The drawing under review shows one solid part. Ordinate dimensions are in mm from its lowest x, y, z. Give positions to 0.01 mm unless a question says otherwise; leave off trailing zeros. Order: outer loops, then holes, each group sorted by start corner. A loop starts at its lowest first (then second) coordinate and runs counter-clockwise, first axis right, second up. Notation, with made-up numbers: (-33.75, 68) -> (-17.75, 68) arc R32 ccw to (-17.75, 98) -> close; hole circle Ø11 at (80.5, 57.5). An arc over 180 degrees is marked (long way). One line per item, written item: value.
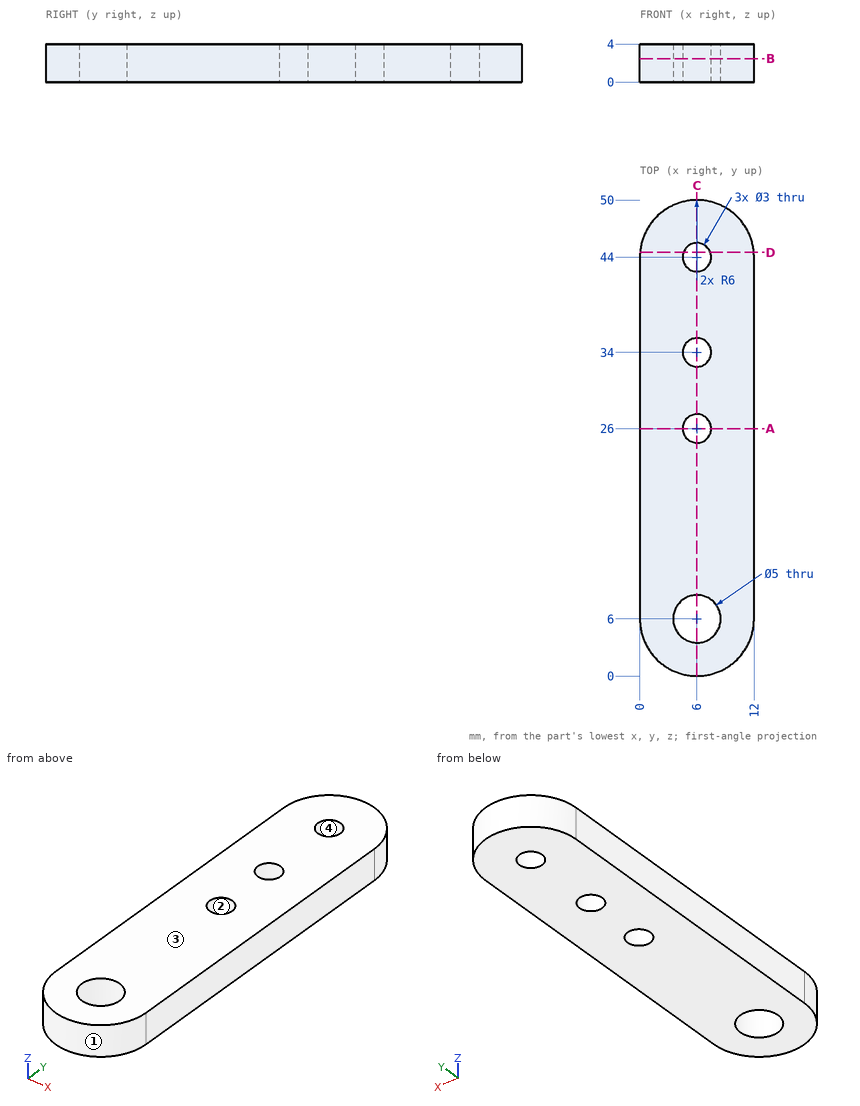
Item 1: Add section D-D on y = 44.5. Give the boundary of the cut face in (x, z), plus the area to 3 significant figures.
Returned:
outline: (0.02, 0) -> (4.59, 0) -> (4.59, 4) -> (0.02, 4) -> close; (7.41, 0) -> (11.98, 0) -> (11.98, 4) -> (7.41, 4) -> close
area: 36.5 mm²
Item 2: Clearance check with a flat-ended pin moving along its axis: P1, Ø4, axis at x = 6, y = 44, coming from the -Z side. State where the tip first meets the part, or that it passes through.
Returned:
P1: z = 0
Item 3: Add section A-A on y = 26. Give the boundary of the cut face in (x, z), plus the area to 3 significant figures.
Returned:
outline: (0, 0) -> (4.5, 0) -> (4.5, 4) -> (0, 4) -> close; (7.5, 0) -> (12, 0) -> (12, 4) -> (7.5, 4) -> close
area: 36.0 mm²
Item 4: Add section B-B on z = 2.45. Give the boundary of the cut face in (x, y).
Returned:
outline: (0, 6) arc R6 ccw to (12, 6) -> (12, 44) arc R6 ccw to (0, 44) -> close; hole circle Ø5 at (6, 6); hole circle Ø3 at (6, 26); hole circle Ø3 at (6, 34); hole circle Ø3 at (6, 44)
Item 5: Draft analysis for pull direction Y (two halves, no side actions). For the marked faces 1, 2, 3 and 4, state which applies: pulls with the +Y half, pulls with the -Y half, needs draft (parallel to the pull), parting line crosses it, or undercut.
Returned:
face 1: pulls with the -Y half
face 2: undercut
face 3: needs draft
face 4: undercut
Item 6: Add section C-C on x = 6. Give the boundary of the cut face in (y, z).
Returned:
outline: (0, 0) -> (3.5, 0) -> (3.5, 4) -> (0, 4) -> close; (8.5, 0) -> (24.5, 0) -> (24.5, 4) -> (8.5, 4) -> close; (27.5, 0) -> (32.5, 0) -> (32.5, 4) -> (27.5, 4) -> close; (35.5, 0) -> (42.5, 0) -> (42.5, 4) -> (35.5, 4) -> close; (45.5, 0) -> (50, 0) -> (50, 4) -> (45.5, 4) -> close
Item 7: To check wall thickness, follow line 1 along Y through (x, z) = (6, 2.7); line 2 along Y through (x, z) = (5, 0.85); line 3 along X through (y, z) = (27, 2.25). State the ranges of each line that lie inside material, in increasing order. Write a range as from..to.
Returned:
line 1: 0..3.5, 8.5..24.5, 27.5..32.5, 35.5..42.5, 45.5..50
line 2: 0.08..3.71, 8.29..24.88, 27.12..32.88, 35.12..42.88, 45.12..49.92
line 3: 0..4.88, 7.12..12
